from build123d import *

# Parameters (mm, degrees)
F0_R      = 11.5
F1_DEPTH  = 6
F3_R      = 11.5
F3_R_2    = 7.75
F4_DEPTH  = 9
F6_R      = 8.5
F7_R      = 11.5
F9_W      = 9.5
F9_H      = 9.5
F10_DEPTH = 10


with BuildPart() as f1:
    # F0 (on Top) → F1 (new body)
    with BuildSketch(Plane.XY):
        Circle(F0_R)
        Polygon((4.494297, 7.47025), (8.716574, -0.15705), (4.222277, -7.6273), (-4.494297, -7.47025), (-8.716574, 0.15705), (-4.222277, 7.6273), align=None, mode=Mode.SUBTRACT)
    extrude(amount=F1_DEPTH)

    # F3 (on offset) → F4 (join)
    with BuildSketch(Plane.XY.offset(6)):
        Circle(F3_R)
        Circle(F3_R_2, mode=Mode.SUBTRACT)
    extrude(amount=F4_DEPTH)

    # F6 (on offset) → F8 section 0
    with BuildSketch(Plane.XY.offset(27)):
        Circle(F6_R)
    # F7 (on face) → F8 section 1
    with BuildSketch(Plane.XY.offset(15)):
        Circle(F7_R)
    loft()

    # F9 (on face) → F10 (cut)
    with BuildSketch(Plane.XY.offset(27)):
        Rectangle(F9_W, F9_H)
    extrude(amount=-F10_DEPTH, mode=Mode.SUBTRACT)

    # F11 (on face) → F12 (revolve, cut)
    with BuildSketch(Plane.XZ.offset(-4.75)):
        with BuildLine():
            ThreePointArc((2.15, 21.75), (1.52028, 23.27028), (0, 23.9))
            Line((0, 23.9), (0, 21.75))
            Line((0, 21.75), (0, 19.6))
            ThreePointArc((0, 19.6), (1.52028, 20.22972), (2.15, 21.75))
        make_face()
    revolve(axis=Axis((0, 4.75, 24.375), (0, 0, -1)), mode=Mode.SUBTRACT)


solid = f1.part
Geometry: final body of the model. Coordinates: model frame, mm. A direction names the side the tool comes from. Round coordinates to 2 decimals unless told otherwise and drop trailing zeros. Order: outer loops, then holes, each group sorted by start corner. A loop starts at its lowest first (then second) coordinate and runs counter-clockwise, first axis right, second up. Notation, with made-up numbers: (53.25, -17) - (98.25, -17) arc R14 cw to (98.25, -7) - close; hole circle Ø10 at (72.25, 2.25). An arc over 180 degrees is marked (long way). Write each question's results on one line, items separated by ' | '.
Item 1: Mould query, pull axis Y, two halves, no side actions, for faces 5 (the flat face through (-4, -7, 6)), 6 (the conical face through (-2.03, -9.13, 23.58)), 7 (the flat face through (0, -6, 27)). Classes: pulls with the +Y half, pulls with the -Y half, needs draft (parallel to the pull), parting line crosses it, or undercut.
Completed:
face 5: undercut | face 6: parting line crosses it | face 7: needs draft
Item 2: Material intervals for line 1 along Y through (x, z) = (0, 11.75); line 2 along Z through (x, y) = (3, -1); line 3 along Z through (x, y) = (7, 2.25), sorted ascending. Write a range as [from, to].
Completed:
line 1: [-11.5, -7.75], [7.75, 11.5] | line 2: [15, 17] | line 3: [15, 27]
Item 3: First-contact query: pin 1 Ø1.5 at (x, z) = (9, 5) entering from +Y; pin 2 Ø10 at (y, z) = (-8, 16.5) entering from +X; pin 3 Ø2 at (x, z) = (4, 13) entering from -Y. Flat tips, straight axial feed; report the tip coordinate or a pass-through.
Completed:
pin 1: y = 8.01 | pin 2: x = 11.04 | pin 3: y = -11.1
Item 4: Reachability of faces 1 (the flat face through (-6.576, -3.71, 2.958)), 2 (the cylindrical face through (-1.009, 7.684, 10.437)), 3 (the flat face through (8, -2, 0)), 4 (the flat face through (4.75, 0, 22)) from +Z, -Z, +X, -X, +Y, -Y: full face, straight path, thin tool, end or side. Return the list, or none.
Completed:
face 1: -Z | face 2: none | face 3: -Z, +X, -X, +Y, -Y | face 4: +Z
Item 5: Section A-A, the plane z = 10.5. Return the cut outline in (x, y).
Completed:
outline: circle Ø23 at (0, 0); hole circle Ø15.5 at (0, 0)
